Can you work these out from the model? Positions are in its coordinate system, mm. A direction names the side the tool comes from. Give positions to 0.01 mm unless a question says otherwise; leave off trailing zeros. Write each loop counter-clockwise with the first axis right and the second up, starting at its lowest first coordinate (ties: lowest second). Pieces come first, ordered by that corner, then holes. Notation, with made-up numbers: M 63,-24.75 L 67,-24.75 A26 ccw 67,14.25 Z; hole C 70.25,16 d4. An arc over 180 degrees is marked long. Write each question's results on one line, items separated by ' | '.
from build123d import *

# Parameters (mm, degrees)
BOSS_EXTRUDE1_DEPTH = 125
CUT_EXTRUDE1_DEPTH  = 402.798830122
CUT_EXTRUDE2_START  = 7.5
CUT_EXTRUDE2_DEPTH  = 110
CUT_EXTRUDE3_START  = 7.5
CUT_EXTRUDE3_DEPTH  = 110
CUT_EXTRUDE4_REACH  = 265.278
SKETCH6_W           = 70.076051312
SKETCH6_H           = 19.92290321
CUT_EXTRUDE5_REACH  = 297.109
SKETCH5_W           = 70
SKETCH5_H           = 20.313376992
CUT_EXTRUDE6_REACH  = 337.806
SKETCH7_W           = 70
SKETCH7_H           = 10
FILLET1_R           = 15
CUT_EXTRUDE7_START  = -125
CUT_EXTRUDE7_DEPTH  = 125
CHAMFER1_START      = 101
CHAMFER1_OUTLINE_W  = 127
CHAMFER1_OUTLINE_H  = 4
CHAMFER1_DEPTH      = 1.291551205


with BuildPart() as part:
    # Sketch1 → Boss-Extrude1 (new body)
    with BuildSketch(Plane(origin=(0, 0, 0), x_dir=(0, 0, -1), z_dir=(1, 0, 0))):
        with BuildLine():
            Line((89.8548345, 121.890508387), (339.8548345, 121.890508387))
            Line((339.8548345, 121.890508387), (339.8548345, 142.698803067))
            Line((339.8548345, 142.698803067), (328.974757131, 148.244473571))
            Line((328.974757131, 148.244473571), (304.07146893, 160.937897169))
            Line((304.07146893, 160.937897169), (291.499350701, 165.900575417))
            ThreePointArc((291.499350701, 165.900575417), (280.939522904, 169.403551358), (270.055923817, 171.711813574))
            Line((270.055923817, 171.711813574), (268.171463935, 172.003048284))
            ThreePointArc((268.171463935, 172.003048284), (254.466056361, 173.586145336), (240.679656072, 174.114879761))
            Line((240.679656072, 174.114879761), (232.021178794, 174.114879761))
            Line((232.021178794, 174.114879761), (204.700095622, 174.114879761))
            Line((204.700095622, 174.114879761), (181.005704906, 172.180643784))
            Line((181.005704906, 172.180643784), (169.793278807, 169.525069181))
            ThreePointArc((169.793278807, 169.525069181), (162.738148163, 167.508293641), (155.897481651, 164.85357451))
            Line((155.897481651, 164.85357451), (139.701268702, 157.697108323))
            ThreePointArc((139.701268702, 157.697108323), (131.522677332, 153.88092637), (123.507487012, 149.732513946))
            Line((123.507487012, 149.732513946), (122.849499947, 149.374661332))
            ThreePointArc((122.849499947, 149.374661332), (105.217865801, 137.440006065), (90.215677989, 122.332230589))
            Line((90.215677989, 122.332230589), (89.8548345, 121.890508387))
        make_face()
    extrude(amount=BOSS_EXTRUDE1_DEPTH)

    # Sketch2 → Cut-Extrude1 (cut, through all)
    with BuildSketch(Plane(origin=(125, 0, 0), x_dir=(0, 0, -1), z_dir=(1, 0, 0))):
        with BuildLine():
            Line((113.475739659, 133.359325966), (201.174236889, 137.018348058))
            Line((201.174236889, 137.018348058), (207.075885424, 168.415118264))
            Line((207.075885424, 168.415118264), (192.666474105, 167.813918061))
            Line((192.666474105, 167.813918061), (190.829871081, 167.73728994))
            ThreePointArc((190.829871081, 167.73728994), (182.233808887, 166.844681368), (173.813252446, 164.899619793))
            Line((173.813252446, 164.899619793), (169.2892062, 163.555605085))
            ThreePointArc((169.2892062, 163.555605085), (160.569837528, 160.5967142), (152.103009161, 156.977979241))
            Line((152.103009161, 156.977979241), (131.888883088, 147.40524948))
            Line((131.888883088, 147.40524948), (120.054289503, 140.950016615))
            ThreePointArc((120.054289503, 140.950016615), (116.601738736, 138.565427019), (113.722697716, 135.512969462))
            Line((113.722697716, 135.512969462), (113.475739659, 135.188837012))
            Line((113.475739659, 135.188837012), (113.475739659, 133.359325966))
        make_face()
        with BuildLine():
            Line((221.003775967, 168.415118264), (218.761149524, 138.906875589))
            Line((218.761149524, 138.906875589), (272.584184163, 138.906875589))
            Line((272.584184163, 138.906875589), (274.383679522, 162.58444611))
            Line((274.383679522, 162.58444611), (267.028526617, 163.966993649))
            Line((267.028526617, 163.966993649), (257.016670223, 165.848921543))
            Line((257.016670223, 165.848921543), (255.744876296, 166.087980551))
            ThreePointArc((255.744876296, 166.087980551), (245.628472921, 167.506912168), (235.424062848, 167.981253005))
            Line((235.424062848, 167.981253005), (234.695600568, 167.981253005))
            Line((234.695600568, 167.981253005), (221.003775967, 168.415118264))
        make_face()
        with BuildLine():
            Line((276.275786009, 160.987395212), (275.646964577, 141.143186512))
            Line((275.646964577, 141.143186512), (283.14790924, 141.143186512))
            Line((283.14790924, 141.143186512), (294.416525801, 147.803376186))
            Line((294.416525801, 147.803376186), (296.046101937, 148.766518919))
            ThreePointArc((296.046101937, 148.766518919), (296.405855365, 149.13182216), (296.537289859, 149.627396535))
            Line((296.537289859, 149.627396535), (296.537289859, 150.540124257))
            ThreePointArc((296.537289859, 150.540124257), (296.433404588, 150.983946735), (296.143333074, 151.335555977))
            Line((296.143333074, 151.335555977), (294.416525801, 152.651218661))
            Line((294.416525801, 152.651218661), (277.097452917, 160.987395212))
            Line((277.097452917, 160.987395212), (276.275786009, 160.987395212))
        make_face()
    extrude(amount=-CUT_EXTRUDE1_DEPTH, mode=Mode.SUBTRACT)

    # Cut-Extrude2: read off the stored shape, not the designer's step
    # Cut-Extrude2 outline → Cut-Extrude2 (cut)
    with BuildSketch(Plane.YZ.offset(CUT_EXTRUDE2_START)):
        with BuildLine():
            Line((121.890508387, -99.688159251), (121.890508387, -171.289102204))
            Line((121.890508387, -171.289102204), (135.747336393, -170.710957294))
            Line((135.747336393, -170.710957294), (133.359325966, -113.475739659))
            Line((133.359325966, -113.475739659), (135.188837012, -113.475739659))
            Line((135.188837012, -113.475739659), (135.512969462, -113.722697716))
            ThreePointArc((135.512969462, -113.722697716), (138.565427019, -116.601738736), (140.950016615, -120.054289503))
            Line((140.950016615, -120.054289503), (147.40524948, -131.888883088))
            Line((147.40524948, -131.888883088), (156.977979241, -152.103009161))
            ThreePointArc((156.977979241, -152.103009161), (160.5967142, -160.569837528), (163.555605085, -169.2892062))
            Line((163.555605085, -169.2892062), (163.632345036, -169.547518172))
            Line((163.632345036, -169.547518172), (169.408178174, -169.306534555))
            ThreePointArc((169.408178174, -169.306534555), (167.428165725, -162.501028912), (164.85357451, -155.897481651))
            Line((164.85357451, -155.897481651), (157.697108323, -139.701268702))
            ThreePointArc((157.697108323, -139.701268702), (153.88092637, -131.522677332), (149.732513946, -123.507487012))
            Line((149.732513946, -123.507487012), (149.374661332, -122.849499947))
            ThreePointArc((149.374661332, -122.849499947), (141.537958861, -110.480020928), (132.127738515, -99.261033903))
            Line((132.127738515, -99.261033903), (121.890508387, -99.688159251))
        make_face()
    extrude(amount=CUT_EXTRUDE2_DEPTH, mode=Mode.SUBTRACT)

    # Cut-Extrude3: read off the stored shape, not the designer's step
    # Cut-Extrude3 outline → Cut-Extrude3 (cut)
    with BuildSketch(Plane.YZ.offset(CUT_EXTRUDE3_START)):
        with BuildLine():
            Line((121.890508387, -291.499350701), (121.890508387, -333.35633566))
            Line((121.890508387, -333.35633566), (146.011144709, -333.35633566))
            Line((146.011144709, -333.35633566), (160.937897169, -304.07146893))
            Line((160.937897169, -304.07146893), (165.900575417, -291.499350701))
            Line((165.900575417, -291.499350701), (154.055340396, -291.499350701))
            Line((154.055340396, -291.499350701), (152.651218661, -294.416525801))
            Line((152.651218661, -294.416525801), (151.335555977, -296.143333074))
            ThreePointArc((151.335555977, -296.143333074), (150.983946735, -296.433404588), (150.540124257, -296.537289859))
            Line((150.540124257, -296.537289859), (149.627396535, -296.537289859))
            ThreePointArc((149.627396535, -296.537289859), (149.13182216, -296.405855365), (148.766518919, -296.046101937))
            Line((148.766518919, -296.046101937), (146.079212499, -291.499350701))
            Line((146.079212499, -291.499350701), (121.890508387, -291.499350701))
        make_face()
    extrude(amount=CUT_EXTRUDE3_DEPTH, mode=Mode.SUBTRACT)

    # Cut-Extrude4: up to this plane
    cut_extrude4_end = Plane(origin=(0, 137.018348058, -201.174236889), z_dir=(0, -0.18473466771426061, -0.9827884322398701))
    # Sketch6 → Cut-Extrude4 (cut, up to the surface)
    with BuildSketch(Plane(origin=(0, -15.732649467, -207.008545619), x_dir=(-1, 0, 0), z_dir=(0, -0.07578145826840303, -0.9971244509000441)), mode=Mode.PRIVATE) as cut_extrude4_sk1:
        with Locations((-57.714978641, 162.925898332)):
            Rectangle(SKETCH6_W, SKETCH6_H)
    cut_extrude4_tool1 = split(extrude(cut_extrude4_sk1.sketch, amount=-CUT_EXTRUDE4_REACH, mode=Mode.PRIVATE), bisect_by=cut_extrude4_end, keep=Keep.BOTH, mode=Mode.PRIVATE)
    add(cut_extrude4_tool1.solids().sort_by_distance((57.714979, 146.724747, -219.355308))[0], mode=Mode.SUBTRACT)

    # Cut-Extrude5: up to this plane
    cut_extrude5_end = Plane(origin=(0, 168.415118264, -221.003775967), z_dir=(0, 0.075781458268403, 0.997124450900044))
    # Sketch5 → Cut-Extrude5 (cut, up to the surface)
    with BuildSketch(Plane(origin=(0, -31.848196468, -169.432405211), x_dir=(1, 0, 0), z_dir=(0, 0.18473466771426064, 0.9827884322398701)), mode=Mode.PRIVATE) as cut_extrude5_sk1:
        with Locations((57.5, 181.980591777)):
            Rectangle(SKETCH5_W, SKETCH5_H)
    cut_extrude5_tool1 = split(extrude(cut_extrude5_sk1.sketch, amount=-CUT_EXTRUDE5_REACH, mode=Mode.PRIVATE), bisect_by=cut_extrude5_end, keep=Keep.BOTH, mode=Mode.PRIVATE)
    add(cut_extrude5_tool1.solids().sort_by_distance((57.5, 147.000224, -203.050529))[0], mode=Mode.SUBTRACT)

    # Cut-Extrude6: up to this plane
    cut_extrude6_end = Plane(origin=(125, 121.890508387, -89.8548345), z_dir=(0, 1, 0))
    # Sketch7 → Cut-Extrude6 (cut, up to the surface)
    with BuildSketch(Plane(origin=(0, 168.866544526, -31.741831678), x_dir=(1, 0, 0), z_dir=(0, 0.9827884322398701, -0.18473466771426067)), mode=Mode.PRIVATE) as cut_extrude6_sk1:
        with Locations((57.5, 177.39967388)):
            Rectangle(SKETCH7_W, SKETCH7_H)
    cut_extrude6_tool1 = split(extrude(cut_extrude6_sk1.sketch, amount=-CUT_EXTRUDE6_REACH, mode=Mode.PRIVATE), bisect_by=cut_extrude6_end, keep=Keep.BOTH, mode=Mode.PRIVATE)
    add(cut_extrude6_tool1.solids().sort_by_distance((57.5, 136.094675, -206.088179))[0], mode=Mode.SUBTRACT)

    # Fillet1
    fillet1_edges = [part.edges().sort_by_distance(p)[0] for p in [
        (125, 132.294655727, -339.8548345),
        (0, 132.294655727, -339.8548345),
    ]]
    fillet(fillet1_edges, radius=FILLET1_R)

    # Sketch14 → Cut-Extrude7 (cut)
    with BuildSketch(Plane(origin=(125, 0, 0), x_dir=(0, 0, -1), z_dir=(1, 0, 0)).offset(CUT_EXTRUDE7_START)):
        Polygon((221.003775967, 168.415118264), (207.075885424, 168.415118264), (199.383679522, 168.094178314), (199.383679522, 127.58444611), (274.383679522, 127.58444611), (274.383679522, 162.58444611), (255.744876296, 166.087980551), (245.628472921, 167.506912168), (235.059831708, 167.981253005), (234.695600568, 167.981253005), align=None)
    extrude(amount=CUT_EXTRUDE7_DEPTH, mode=Mode.SUBTRACT)

    # Chamfer1: read off the stored shape, not the designer's step
    # Chamfer1 outline → Chamfer1 (cut)
    with BuildSketch(Plane(origin=(0, 0, 0), x_dir=(1, 0, 0), z_dir=(0, 0.09991010561593, -0.99499646773032)).offset(CHAMFER1_START)):
        with Locations((62.5, -113)):
            Rectangle(CHAMFER1_OUTLINE_W, CHAMFER1_OUTLINE_H)
    extrude(amount=CHAMFER1_DEPTH, mode=Mode.SUBTRACT)


solid = part.part
Item 1: I want a section at A-A, the plane z = -215. Please give me the cut outline in (x, y), and give its area (3 significant figures).
Geometry says:
outline: M 0,121.89 L 125,121.89 L 125,127.58 L 0,127.58 Z; M 0,168.42 L 125,168.42 L 125,174.11 L 0,174.11 Z | area: 1,420 mm2
Item 2: I'm going to push flat-ended pins straight in: pin 1 (1.5 mm diameter, centred on x = 4.5, y = 134.5, fed in from -Z); pin 2 (5 mm diameter, centred on x = 100.5, y = 162, fed in from -Z); pin 3 (1 mm diameter, centred on x = 4.5, y = 150, fed in from +Z). Where does each tip first touch, or does it pass through?
Geometry says:
pin 1: stops at z = -336.25 | pin 2: stops at z = -291.5 | pin 3: stops at z = -123.08
Item 3: If I drill on line 1 (Z direction, x = 38.5, y = 134.5); line 2 (Y direction, x = 47, z = -240.5); line 3 (Z direction, x = 46, y = 144), over which ranges is the centre line in solid material (lowest first)? Write a range as from..to.
Geometry says:
line 1: z = -339.85..-333.36, -291.5..-274.38, -199.38..-170.76 | line 2: y = 121.89..127.58, 167.86..174.11 | line 3: z = -337.3..-333.36, -291.5..-287.98, -275.74..-274.38
Item 4: I want a section at B-B, the plane y = 125. Please give me the cut outline in (x, z).
Geometry says:
outline: M 0,-324.85 A15 ccw 15,-339.85 L 110,-339.85 A15 ccw 125,-324.85 L 125,-92.47 L 0,-92.47 Z; hole M 7.5,-333.36 L 117.5,-333.36 L 117.5,-291.5 L 7.5,-291.5 Z; hole M 7.5,-171.16 L 117.5,-171.16 L 117.5,-99.56 L 7.5,-99.56 Z; hole M 22.5,-209.09 L 92.5,-209.09 L 92.5,-198.92 L 22.5,-198.92 Z
Item 5: For faces 4 (the face through (62, 160, -291.499)), 5 (the face through (57.01, 124.777, -198.873)), 6 (the face through (121.3, 152.26, -142.14)), 7 (the face through (61.73, 166.48, -169.43)), which set-ups out of +Z, -Z, +X, -X, +Y, -Y let a thin tool reach every point of the face, with its end or its side?
Geometry says:
face 4: -Z, +Y, -Y | face 5: -Y | face 6: +X, -X | face 7: +Z, -Y
Item 6: I want a section at C-C, the plane z = -135.5. Please give me the cut outline in (x, y).
Geometry says:
outline: M 0,121.89 L 7.5,121.89 L 7.5,134.28 L 0,134.28 Z; M 0,149.12 L 7.5,149.12 L 7.5,155.79 L 0,155.79 Z; M 117.5,121.89 L 125,121.89 L 125,134.28 L 117.5,134.28 Z; M 117.5,149.12 L 125,149.12 L 125,155.79 L 117.5,155.79 Z
Item 7: Thinking about a two-plate mould opening in Z: for faces 1 (the face through (61.73, 128.722, -171.004)), 2 (the face through (3.7, 153.94, -131.64)), 3 (the face through (121.198, 163.384, -297.873)), which applies, +Z half, -Z half, draft (parallel to the pull), parting line (faces both ways), or undercut?
Geometry says:
face 1: undercut | face 2: +Z half | face 3: -Z half
Item 8: I want a section at D-D, the plane x = 103. Give the number of separate pieces and of enclosed holes in the cut face, and give its area (3 significant figures).
Geometry says:
separate pieces: 3 | enclosed holes: 0 | area: 2,250 mm2
